For this review, take the finished solid that the model builds, in its own axes (mm). A direction names the side the tool comes from. Coordinates: 2 decimals unless noted, no trailing zeros. Loops run counter-clockwise (first coordinate to the right, second up) from the corner with the lowest first, then second, coordinate; pieces in that order, holes last. Notation, with made-up numbers: M 67.5,40 L 119.5,40 A23 ccw 119.5,73 Z; hole C -36,49 d2. An arc over 180 degrees is marked long. Answer as a JSON object with one key per item and string values. Group by question number.
Item 1: Insertion check: pin 1 (6 mm diameter, centred on x = 3.5, z = -13, fed in from -Y); pin 2 (1.6 mm diameter, centred on x = -20, z = 29, fed in from +Y); pin 3 (1 mm diameter, centred on x = -3, z = -7.5, fed in from +Y). Each pin has a flat end and moves straight along its axis. Give the tip position at first contact, or say it passes through.
Item 2: Add section B-B (x = 9.5). State the section outline as (y, z) points (3 decimals), then the cut area to 3 significant figures.
Item 3: Add section A-A (y = 19.5). State the section outline as (x, z) points (3 decimals), then the cut area to 3 significant figures.
Item 4: Tool access review of faces 1 (the face through (21.1, 1.5, 1)), 2 (the face through (25.5, 13, -29.1)), 3 (the face through (35.992, -2, -19)), 4 (the face through (-36.398, -2, 19)): name each direction out of +Z, -Z, +X, -X, +Y, -Y from which nothing blocks a thin tool from reaching the whole face with its end or side.
Item 5: Wall thickness on L1, parallel to Z at x = -27.94, y = 1.15 (3 decimals); L2, parallel to Z at x = -18, y = 8.5 (3 decimals); L3, parallel to X at y = 4.5, z = 4: over which ranges is each line inside the solid? List them lowest first. Write a range as from..to.
Item 6: Mouldability with a two-part tool opening along Z and no side actions: class faces 5 (the face through (-28.148, 0.761, 17.717)), 6 (the face through (-25.5, 13, 29.1)) as +Z half, -Z half, draft (parallel to the pull), parting line (faces both ways), or undercut.
from build123d import *

# Parameters (mm, degrees)
SKETCH1_W                 = 77.724
SKETCH1_H                 = 59.69
BOSS_EXTRUDE1_DEPTH       = 21.59
SKETCH2_W                 = 0.4064
SKETCH2_H                 = 1.5748
BOSS_EXTRUDE2_DEPTH       = 3.175
SKETCH3_W                 = 0.4064
SKETCH3_H                 = 1.5748
BOSS_EXTRUDE3_DEPTH       = 3.175
SKETCH4_W                 = 0.4064
SKETCH4_H                 = 1.5748
BOSS_EXTRUDE4_DEPTH       = 3.175
SKETCH5_W                 = 0.4064
SKETCH5_H                 = 1.5748
BOSS_EXTRUDE5_DEPTH       = 3.175
SKETCH6_W                 = 0.4064
SKETCH6_H                 = 1.5748
BOSS_EXTRUDE6_DEPTH       = 3.175
SKETCH7_W                 = 0.4064
SKETCH7_H                 = 1.5748
BOSS_EXTRUDE7_DEPTH       = 3.175
F_4_CLEARANCE_HOLE1_D     = 3.2004
F_4_CLEARANCE_HOLE1_DEPTH = 5.08
SHELL1_START              = 1.5
SHELL1_OUTLINE_W          = 74.724
SHELL1_OUTLINE_H          = 56.69
SHELL1_OUTLINE_R          = 3.1002
SHELL1_DEPTH              = 20.09
SHELL1_START_2            = 6.58
SHELL1_2_OUTLINE_R        = 3.1002
SHELL1_2_DEPTH            = 15.01
FILLET1_R                 = 5
CUT_EXTRUDE3_DEPTH        = 75.426334345
SKETCH11_W                = 74.724
SKETCH11_H                = 46.69
CUT_EXTRUDE4_DEPTH        = 53.958353156
SKETCH12_W                = 74.724
SKETCH12_H                = 1
BOSS_EXTRUDE8_DEPTH       = 15.5
CUT_EXTRUDE5_REACH        = 61.182
FILLET2_R                 = 3
SKETCH14_R                = 1.905686258
CUT_EXTRUDE6_DEPTH        = 0.2
LPATTERN1_COUNT           = 3
LPATTERN1_PITCH           = 17.5


# Read off the part's stored shape, not the designer's step: Shell1
with BuildPart() as part:
    # Sketch1 → Boss-Extrude1 (new body)
    with BuildSketch(Plane.XZ):
        Rectangle(SKETCH1_W, SKETCH1_H)
    extrude(amount=-BOSS_EXTRUDE1_DEPTH)

    # Sketch2 → Boss-Extrude2 (add)
    with BuildSketch(Plane.XZ):
        with Locations((-36.195, 0)):
            Rectangle(SKETCH2_W, SKETCH2_H)
    extrude(amount=BOSS_EXTRUDE2_DEPTH)

    # Sketch3 → Boss-Extrude3 (add)
    with BuildSketch(Plane.XZ):
        with Locations((36.195, 0)):
            Rectangle(SKETCH3_W, SKETCH3_H)
    extrude(amount=BOSS_EXTRUDE3_DEPTH)

    # Sketch4 → Boss-Extrude4 (add)
    with BuildSketch(Plane.XZ):
        with Locations((-36.195, 19.304)):
            Rectangle(SKETCH4_W, SKETCH4_H)
    extrude(amount=BOSS_EXTRUDE4_DEPTH)

    # Sketch5 → Boss-Extrude5 (add)
    with BuildSketch(Plane.XZ):
        with Locations((36.195, 19.304)):
            Rectangle(SKETCH5_W, SKETCH5_H)
    extrude(amount=BOSS_EXTRUDE5_DEPTH)

    # Sketch6 → Boss-Extrude6 (add)
    with BuildSketch(Plane.XZ):
        with Locations((36.195, -19.304)):
            Rectangle(SKETCH6_W, SKETCH6_H)
    extrude(amount=BOSS_EXTRUDE6_DEPTH)

    # Sketch7 → Boss-Extrude7 (add)
    with BuildSketch(Plane.XZ):
        with Locations((-36.195, -19.304)):
            Rectangle(SKETCH7_W, SKETCH7_H)
    extrude(amount=BOSS_EXTRUDE7_DEPTH)

    # #4 Clearance Hole1
    with Locations(Plane(origin=(0, 0, 0), x_dir=(-1, 0, 0), z_dir=(0, -1, 0))):
        with Locations((27.94, 19.304), (27.94, 0), (-27.686, 19.304), (-27.686, 0), (-27.686, -19.304), (27.94, -19.304)):
            Hole(F_4_CLEARANCE_HOLE1_D / 2, depth=F_4_CLEARANCE_HOLE1_DEPTH)

    # Shell1 outline → Shell1 (cut)
    with BuildSketch(Plane(origin=(0, 0, 0), x_dir=(1, 0, 0), z_dir=(0, 1, 0)).offset(SHELL1_START)):
        Rectangle(SHELL1_OUTLINE_W, SHELL1_OUTLINE_H)
        with Locations((-27.94, -19.304)):
            Circle(SHELL1_OUTLINE_R, mode=Mode.SUBTRACT)
        with Locations((-27.94, 0)):
            Circle(SHELL1_OUTLINE_R, mode=Mode.SUBTRACT)
        with Locations((27.686, -19.304)):
            Circle(SHELL1_OUTLINE_R, mode=Mode.SUBTRACT)
        with Locations((27.686, 0)):
            Circle(SHELL1_OUTLINE_R, mode=Mode.SUBTRACT)
        with Locations((-27.94, 19.304)):
            Circle(SHELL1_OUTLINE_R, mode=Mode.SUBTRACT)
        with Locations((27.686, 19.304)):
            Circle(SHELL1_OUTLINE_R, mode=Mode.SUBTRACT)
    extrude(amount=SHELL1_DEPTH, mode=Mode.SUBTRACT)

    # Shell1 2 outline → Shell1 2 (cut)
    with BuildSketch(Plane(origin=(0, 0, 0), x_dir=(1, 0, 0), z_dir=(0, 1, 0)).offset(SHELL1_START_2)):
        with Locations((-27.94, -19.304)):
            Circle(SHELL1_2_OUTLINE_R)
        with Locations((27.686, -19.304)):
            Circle(SHELL1_2_OUTLINE_R)
        with Locations((27.686, 0)):
            Circle(SHELL1_2_OUTLINE_R)
        with Locations((27.686, 19.304)):
            Circle(SHELL1_2_OUTLINE_R)
        with Locations((-27.94, 0)):
            Circle(SHELL1_2_OUTLINE_R)
        with Locations((-27.94, 19.304)):
            Circle(SHELL1_2_OUTLINE_R)
    extrude(amount=SHELL1_2_DEPTH, mode=Mode.SUBTRACT)

    # Fillet1
    fillet1_edges = [part.edges().sort_by_distance(p)[0] for p in [
        (0, 1.5, 28.345),
        (0, 1.5, -28.345),
    ]]
    fillet(fillet1_edges, radius=FILLET1_R)

    # Sketch10 → Cut-Extrude3 (cut, through all)
    with BuildSketch(Plane(origin=(0, 0, -29.845), x_dir=(-1, 0, 0), z_dir=(0, 0, -1))):
        Polygon((0, 7), (12.75, 7), (12.75, 11), (23.5, 11), (27.5, 15), (37.362, 15), (37.362, 21.59), (0, 21.59), align=None)
    cut_extrude3 = extrude(amount=-CUT_EXTRUDE3_DEPTH, mode=Mode.SUBTRACT)

    # Mirror1: Cut-Extrude3 across plane
    add(cut_extrude3.mirror(Plane(origin=(0, 0, 0), x_dir=(0, 0, 1), z_dir=(1, 0, 0))), mode=Mode.SUBTRACT)

    # Sketch11 → Cut-Extrude4 (cut, through all)
    with BuildSketch(Plane(origin=(0, 1.5, 0), x_dir=(1, 0, 0), z_dir=(0, 1, 0))):
        Rectangle(SKETCH11_W, SKETCH11_H)
    extrude(amount=CUT_EXTRUDE4_DEPTH, mode=Mode.SUBTRACT)

    # Sketch12 → Boss-Extrude8 (add)
    with BuildSketch(Plane(origin=(0, 1.5, 0), x_dir=(1, 0, 0), z_dir=(0, 1, 0))):
        with Locations((0, 9.72)):
            Rectangle(SKETCH12_W, SKETCH12_H)
    boss_extrude8 = extrude(amount=BOSS_EXTRUDE8_DEPTH)

    # Sketch13 → Cut-Extrude5 (cut, up to next)
    with BuildSketch(Plane.XY.offset(-9.22), mode=Mode.PRIVATE) as cut_extrude5_sk1:
        Polygon((-32.5, 17), (-28, 11.5), (28, 11.5), (32.5, 17), align=None)
    cut_extrude5_tool1 = extrude(cut_extrude5_sk1.sketch, amount=-CUT_EXTRUDE5_REACH, mode=Mode.PRIVATE) & part.part
    cut_extrude5 = cut_extrude5_tool1.solids().sort_by_distance((0, 14.318182, -9.22))[0]
    add(cut_extrude5, mode=Mode.SUBTRACT)

    # Mirror2: Boss-Extrude8, Cut-Extrude5 across plane
    add(boss_extrude8.mirror(Plane.XY))
    add(cut_extrude5.mirror(Plane.XY), mode=Mode.SUBTRACT)

    # Fillet2
    fillet2_edges = [part.edges().sort_by_distance(p)[0] for p in [
        (-27.5, 15, 29.095),
        (-27.5, 15, -29.095),
        (-23.5, 11, 29.095),
        (-23.5, 11, -29.095),
        (-12.75, 11, 29.095),
        (-12.75, 11, -29.095),
        (-37.362, 15, 29.095),
        (-37.362, 15, -29.095),
        (12.75, 11, 29.095),
        (12.75, 11, -29.095),
        (23.5, 11, 29.095),
        (23.5, 11, -29.095),
        (37.362, 15, 29.095),
        (37.362, 15, -29.095),
        (27.5, 15, 29.095),
        (27.5, 15, -29.095),
        (-32.5, 17, -9.72),
        (32.5, 17, -9.72),
        (28, 11.5, -9.72),
        (-28, 11.5, -9.72),
        (32.5, 17, 9.72),
        (-32.5, 17, 9.72),
        (-28, 11.5, 9.72),
        (28, 11.5, 9.72),
    ]]
    fillet(fillet2_edges, radius=FILLET2_R)

    # Sketch14 → Cut-Extrude6 (cut)
    with BuildSketch(Plane(origin=(0, 1.5, 0), x_dir=(1, 0, 0), z_dir=(0, 1, 0))):
        with Locations(Location((21.159931599, 16.535374869, 0), (0, 0, 270))):
            Circle(SKETCH14_R)
        Polygon((20.972468472, 16.692908218), (20.972468472, 17.7249595), (21.286571036, 17.7249595), (21.286571036, 16.692908218), (22.318622318, 16.692908218), (22.318622318, 16.378805654), (21.286571036, 16.378805654), (21.286571036, 15.346754372), (20.972468472, 15.346754372), (20.972468472, 16.378805654), (19.94041719, 16.378805654), (19.94041719, 16.692908218), align=None, mode=Mode.SUBTRACT)
    cut_extrude6 = extrude(amount=-CUT_EXTRUDE6_DEPTH, mode=Mode.SUBTRACT)

    # LPattern1: Cut-Extrude6 ×3
    with Locations(*[(0, 0, i * LPATTERN1_PITCH) for i in range(1, LPATTERN1_COUNT)]):
        add(cut_extrude6, mode=Mode.SUBTRACT)


solid = part.part
From the geometry:
{
 "1": {"pin 1": "stops at y = 0", "pin 2": "stops at y = 11", "pin 3": "stops at y = 1.5"},
 "2": {"outline": "M 0,-29.845 L 7,-29.845 L 7,-28.345 L 6.5,-28.345 A5 cw 1.5,-23.345 L 1.5,-10.22 L 11.5,-10.22 L 11.5,-9.22 L 1.5,-9.22 L 1.5,9.22 L 11.5,9.22 L 11.5,10.22 L 1.5,10.22 L 1.5,23.345 A5 cw 6.5,28.345 L 7,28.345 L 7,29.845 L 0,29.845 Z", "area": "137 mm²"},
 "3": {"outline": "M -38.862,-29.845 L -37.362,-29.845 L -37.362,29.845 L -38.862,29.845 Z; M 37.362,-29.845 L 38.862,-29.845 L 38.862,29.845 L 37.362,29.845 Z", "area": "179 mm²"},
 "4": {"face 1": "+Y", "face 2": "+Z, -Z, +Y", "face 3": "+Z, -Z, -Y", "face 4": "+Z, -Z, -X, -Y"},
 "5": {"L1": "z = -29.845..-20.904, -17.704..-1.6, 1.6..17.704, 20.904..29.845", "L2": "z = -29.845..-28.345, -10.22..-9.22, 9.22..10.22, 28.345..29.845", "L3": "x = -38.86..-37.36, 37.36..38.86"},
 "6": {"face 5": "undercut", "face 6": "draft"}
}
